Autodesk Inventor part; units mm, degrees
ref_plane "YZ Plane" through (0, 0, 0) normal (1, 0, 0) x (0, 1, 0)
ref_plane "XZ Plane" through (0, 0, 0) normal (0, 1, 0) x (-1, 0, 0)
ref_plane "XY Plane" through (0, 0, 0) normal (0, 0, 1) x (1, 0, 0)
sketch "Sketch1" plane through (0, 0, 0) normal (0, 0, 1) x (1, 0, 0)
  line L0 (0, 0) -> (300, 0)
  line L1 (300, 0) -> (300, 200)
  line L2 (300, 200) -> (0, 200)
  line L3 (0, 200) -> (0, 0)
  line L4 (10, 10) -> (290, 10)
  line L5 (290, 10) -> (290, 190)
  line L6 (290, 190) -> (10, 190)
  line L7 (10, 190) -> (10, 10)
  line L8 (13.75, 13.75) -> (286.25, 13.75)
  line L9 (286.25, 13.75) -> (286.25, 186.25)
  line L10 (286.25, 186.25) -> (13.75, 186.25)
  line L11 (13.75, 186.25) -> (13.75, 13.75)
  line L12 (38.75, 190) -> (68.5, 190)
  line L13 (68.5, 190) -> (68.5, 186.25)
  line L14 (68.5, 186.25) -> (38.75, 186.25)
  line L15 (38.75, 186.25) -> (38.75, 190)
  line L16 (10, 161.25) -> (13.75, 161.25)
  line L17 (13.75, 161.25) -> (13.75, 131.5)
  line L18 (13.75, 131.5) -> (10, 131.5)
  line L19 (10, 131.5) -> (10, 161.25)
  line L20 (0, 0) -> (150, 0)
  line L21 (150, 0) -> (150, 100)
  line L22 (150, 100) -> (0, 100)
  line L23 (0, 100) -> (0, 0)
  line L24 (38.75, 10) -> (68.5, 10)
  line L25 (68.5, 10) -> (68.5, 13.75)
  line L26 (68.5, 13.75) -> (38.75, 13.75)
  line L27 (38.75, 13.75) -> (38.75, 10)
  line L28 (10, 38.75) -> (13.75, 38.75)
  line L29 (13.75, 38.75) -> (13.75, 68.5)
  line L30 (13.75, 68.5) -> (10, 68.5)
  line L31 (10, 68.5) -> (10, 38.75)
  line L32 (150, 200) -> (150, 100)
  line L33 (300, 200) -> (300, 0)
  line L34 (261.25, 190) -> (231.5, 190)
  line L35 (231.5, 190) -> (231.5, 186.25)
  line L36 (231.5, 186.25) -> (261.25, 186.25)
  line L37 (261.25, 186.25) -> (261.25, 190)
  line L38 (290, 161.25) -> (286.25, 161.25)
  line L39 (286.25, 161.25) -> (286.25, 131.5)
  line L40 (286.25, 131.5) -> (290, 131.5)
  line L41 (290, 131.5) -> (290, 161.25)
  line L42 (300, 100) -> (300, 0)
  line L43 (261.25, 13.75) -> (261.25, 10)
  line L44 (231.5, 10) -> (231.5, 13.75)
  line L45 (231.5, 13.75) -> (261.25, 13.75)
  line L46 (261.25, 10) -> (231.5, 10)
  line L47 (286.25, 68.5) -> (290, 68.5)
  line L48 (290, 38.75) -> (286.25, 38.75)
  line L49 (290, 68.5) -> (290, 38.75)
  line L50 (286.25, 38.75) -> (286.25, 68.5)
  point P0 (13.75, 161.25)
  point P1 (10, 131.5)
  point P2 (10, 68.5)
  point P3 (13.75, 68.5)
  point P4 (13.75, 38.75)
  point P5 (10, 38.75)
  point P6 (68.5, 13.75)
  point P7 (68.5, 10)
  point P8 (38.75, 10)
  point P9 (38.75, 13.75)
  point P10 (231.5, 186.25)
  point P11 (231.5, 190)
  point P12 (261.25, 190)
  point P13 (261.25, 186.25)
  point P14 (286.25, 131.5)
  point P15 (286.25, 161.25)
  point P16 (290, 161.25)
  point P17 (261.25, 13.75)
  point P18 (261.25, 10)
  point P19 (231.5, 10)
  point P20 (231.5, 13.75)
  point P21 (286.25, 68.5)
  point P22 (286.25, 38.75)
  point P23 (68.5, 190)
  dimension "d0" = 300
  dimension "d1" = 200
  dimension "d2" = 280
  dimension "d3" = 180
  dimension "d4" = 10
  dimension "d5" = 10
  dimension "d6" = 3.75
  dimension "d7" = 3.75
  dimension "d8" = 3.75
  dimension "d9" = 3.75
  dimension "d10" = 25
  dimension "d11" = 29.75
  dimension "d12" = 29.75
  dimension "d13" = 25
  dimension "d14" = 100
  dimension "d15" = 150
extrude "Extrusion1" add sketch "Sketch1" along normal blind 4 contours L3 L22 L7 L4 L21 L0 | L21 L4 L5 L6 L32 L2 L1 L0 | L3 L2 L32 L6 L7 L22 | L21 L8 L44 L4 | L4 L25 L8 L21 | L22 L11 L30 L7 | L7 L18 L11 L22 | L21 L32 L10 L9 L8 | L8 L11 L22 L21 | L11 L10 L32 L22 | L4 L7 L28 L11 L8 L27 | L43 L8 L9 L48 L5 L4 | L32 L10 L13 L6 | L6 L35 L10 L32 | L7 L6 L15 L10 L11 L16 | L6 L5 L38 L9 L10 L37 | L47 L9 L40 L5
sketch "Sketch2" plane through (0, 0, 4) normal (0, 0, 1) x (1, 0, 0)
  line L0 (0, 0) -> (60, 0)
  line L1 (60, 0) -> (60, 100)
  line L2 (60, 100) -> (0, 100)
  line L3 (0, 100) -> (0, 0)
  circle A0 centre (60, 100) radius 28
  circle A1 centre (85, 125) radius 2.1
  circle A2 centre (35, 125) radius 2.1
  circle A3 centre (35, 75) radius 2.1
  circle A4 centre (85, 75) radius 2.1
  dimension "d16" = 4
  dimension "d18" = 100
  dimension "d19" = 60
  dimension "d20" = 56
  dimension "d21" = 4.2
  dimension "d22" = 4.2
  dimension "d23" = 4.2
  dimension "d24" = 4.2
  dimension "d25" = 50
  dimension "d26" = 50
  dimension "d27" = 50
  dimension "d28" = 50
  dimension "d29" = 25
  dimension "d30" = 25
  dimension "d31" = 25
  dimension "d32" = 25
extrude "Extrusion2" cut sketch "Sketch2" against normal blind 10 contours A0 L2 L1 | L1 L2 A0 | A1 | A2 | A3 | A4
sketch "Sketch5" plane through (0, 0, 4) normal (0, 0, 1) x (1, 0, 0)
  line L0 (103.75, 114.875) -> (107.5, 114.875)
  line L1 (107.5, 114.875) -> (107.5, 85.125)
  line L2 (107.5, 85.125) -> (103.75, 85.125)
  line L3 (103.75, 85.125) -> (103.75, 114.875)
  line L4 (13.75, 68.5) -> (13.75, 38.75)
  line L5 (0, 0) -> (300, 0)
  point P0 (107.5, 100)
  dimension "d53" = 3.75
  dimension "d54" = 29.75
  dimension "d55" = 90
  dimension "d56" = 100
extrude "Extrusion5" cut sketch "Sketch5" against normal through all
sketch "Sketch6" plane through (0, 0, 4) normal (0, 0, 1) x (1, 0, 0)
  line L0 (286.25, 38.75) -> (286.25, 68.5)
  line L1 (290, 38.75) -> (286.25, 38.75)
  line L2 (286.25, 38.75) -> (286.25, 68.5)
  line L3 (286.25, 68.5) -> (290, 68.5)
  line L4 (290, 68.5) -> (290, 38.75)
  line L5 (286.25, 131.5) -> (286.25, 161.25)
  line L6 (290, 131.5) -> (286.25, 131.5)
  line L7 (286.25, 131.5) -> (286.25, 161.25)
  line L8 (286.25, 161.25) -> (290, 161.25)
  line L9 (290, 161.25) -> (290, 131.5)
  line L10 (290, 68.5) -> (290, 38.75)
  line L11 (290, 53.5) -> (286.25, 53.5)
  line L12 (286.25, 53.5) -> (286.25, 113.5)
  line L13 (286.25, 113.5) -> (290, 113.5)
  line L14 (290, 113.5) -> (290, 53.5)
  point P0 (0, 0)
  dimension "d59" = 60
  dimension "d60" = 15
extrude "Extrusion6" add sketch "Sketch6" against normal blind 4 contours L0 L11 L4 L1 | L5 L8 L9 L6
extrude "Extrusion7" cut sketch "Sketch6" against normal blind 4 contours L0 L3 L4 L11 | L12 L13 L14 L3
sketch "Sketch7" plane through (0, 0, 4) normal (0, 0, 1) x (1, 0, 0)
  line L0 (261.25, 186.25) -> (231.5, 186.25)
  line L1 (261.25, 186.25) -> (201.25, 186.25)
  line L2 (201.25, 186.25) -> (201.25, 190)
  line L3 (201.25, 190) -> (261.25, 190)
  line L4 (261.25, 190) -> (261.25, 186.25)
  line L5 (231.5, 190) -> (261.25, 190)
  line L6 (261.25, 13.75) -> (261.25, 10)
  line L7 (261.25, 10) -> (201.25, 10)
  line L8 (201.25, 10) -> (201.25, 13.75)
  line L9 (201.25, 13.75) -> (261.25, 13.75)
  line L10 (261.25, 13.75) -> (261.25, 10)
  point P0 (0, 0)
  dimension "d65" = 0
  dimension "d66" = 60
  dimension "d67" = 3.75
  dimension "d68" = 60
extrude "Extrusion8" cut sketch "Sketch7" against normal through all
sketch "Sketch8" plane through (0, 0, 4) normal (0, 0, 1) x (1, 0, 0)
  line L0 (86, 106.25) -> (92, 106.25)
  line L1 (92, 106.25) -> (92, 93.75)
  line L2 (92, 93.75) -> (86, 93.75)
  line L3 (86, 93.75) -> (86, 106.25)
  line L4 (0, 200) -> (0, 0)
  line L5 (0, 0) -> (300, 0)
  dimension "d73" = 6
  dimension "d74" = 12.5
  dimension "d75" = 92
  dimension "d76" = 93.75
extrude "Extrusion9" cut sketch "Sketch8" against normal through all
properties part number "bovenstuk_8AUG"
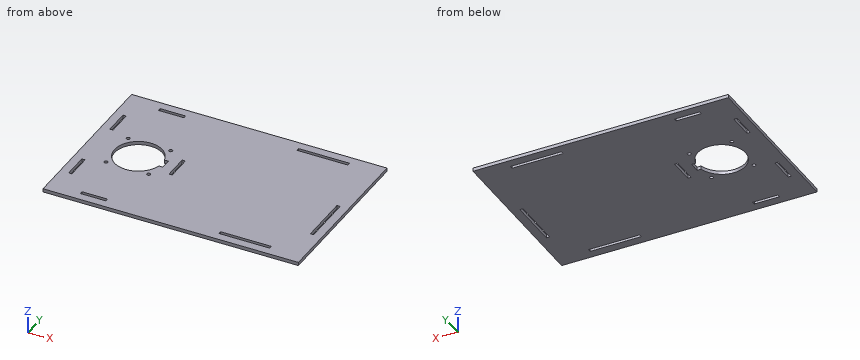
Build history of the part. All positions in model axes, mm. Give positions to 0.01 mm unless a question says otherwise; leave off trailing zeros. Order: outer loops, then holes, each group sorted by start corner. A loop starts at its lowest first (then second) coordinate and runs counter-clockwise, first axis right, second up. Notation, with made-up numbers: M 10,34 L 49,34 A26 ccw 49,53 Z; hole C -5,9 d3. An arc over 180 degrees is marked long. Put each result on its own line as item: value.
Item 1: Slice it at A-A, the plane x = 220. Write the cut outline in (y, z).
From the geometry:
outline: M 0,0 L 10,0 L 10,4 L 0,4 Z; M 13.75,0 L 186.25,0 L 186.25,4 L 13.75,4 Z; M 190,0 L 200,0 L 200,4 L 190,4 Z
Item 2: Slice it at C-C, the plane x = 47.5. Write the cut outline in (y, z), plus the area to 3 significant figures.
From the geometry:
outline: M 0,0 L 10,0 L 10,4 L 0,4 Z; M 13.75,0 L 74.95,0 L 74.95,4 L 13.75,4 Z; M 125.05,0 L 186.25,0 L 186.25,4 L 125.05,4 Z; M 190,0 L 200,0 L 200,4 L 190,4 Z
area: 570 mm2
Item 3: Slice it at D-D, the plane z = 3.35. Give the number of separate pieces and of enclosed holes in the cut face, plus the area to 3 significant figures.
From the geometry:
separate pieces: 1
enclosed holes: 13
area: 56,200 mm2
Item 4: Probe line 1 (Y direction, x = 60, z = 3.15); line 2 (Y direction, x = 255, z = 3); line 3 (X direction, y = 100, z = 2.35). List the from-to ranges inside material, lowest first. Write a range as [from, to].
From the geometry:
line 1: y = [0, 10], [13.75, 72], [128, 186.25], [190, 200]
line 2: y = [0, 10], [13.75, 186.25], [190, 200]
line 3: x = [0, 32], [92, 103.75], [107.5, 286.25], [290, 300]
Item 5: Slice it at B-B, the plane y = 100. Write the cut outline in (x, z), plus the area to 3 significant figures.
From the geometry:
outline: M 0,0 L 32,0 L 32,4 L 0,4 Z; M 92,0 L 103.75,0 L 103.75,4 L 92,4 Z; M 107.5,0 L 286.25,0 L 286.25,4 L 107.5,4 Z; M 290,0 L 300,0 L 300,4 L 290,4 Z
area: 930 mm2
